Could you check a few things on this model? Use its own coordinates, in mm. Face numbers are marked on the shaded views. Give positions to 0.01 mm unless a question says otherwise; leave off trailing zeros. Write each question's results on one line, items separated by ' | '. Start each with the question number.
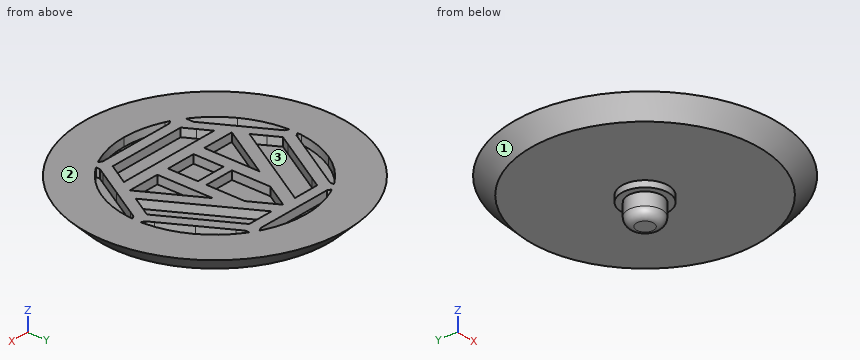
from build123d import *

# Parameters (mm, degrees)
F0_R     = 32
F1_DEPTH = 4
F3_R     = 5.5
F3_R_2   = 4.025
F4_DEPTH = 1.5
F5_DEPTH = 6.5
F7_DEPTH = 2
F8_R     = 2


# Not quite as in the source:
# - a fillet or chamfer that OpenCascade refuses, or shapes differently, is made with other operations: its cross-section is extruded or revolved along the edge and cut away or added


with BuildPart() as f1:
    # F0 (on Top) → F1 (new body)
    with BuildSketch(Plane.XY):
        Circle(F0_R)
    extrude(amount=F1_DEPTH)

    # F2: chamfer of 5 on 1 edges, made by hand

    # F2_s1 → F2_t2 (revolve, cut)
    with BuildSketch(Plane.XZ):
        Polygon((32, 5), (27, 0), (32, 0), align=None)
    revolve(axis=Axis((0, 0, 0), (0, 0, 1)), mode=Mode.SUBTRACT)

    # F3 (on face) → F4 (join)
    with BuildSketch(Plane(origin=(0, 0, 0), x_dir=(1, 0, 0), z_dir=(0, 0, -1))):
        Circle(F3_R)
        Circle(F3_R_2, mode=Mode.SUBTRACT)
    extrude(amount=F4_DEPTH)

    # F3 (on face) → F5 (join)
    with BuildSketch(Plane(origin=(0, 0, 0), x_dir=(1, 0, 0), z_dir=(0, 0, -1))):
        Circle(F3_R_2)
    extrude(amount=F5_DEPTH)

    # F6 (on face) → F7 (cut)
    with BuildSketch(Plane.XY.offset(4)):
        with BuildLine():
            Line((16.237976321, -9.375), (18.75, -10.8253175473))
            ThreePointArc((18.75, -10.8253175473), (20.6335015486, -6.5580952909), (21.5593108924, -1.9864827825))
            Line((21.5593108924, -1.9864827825), (19.9759526419, -2.9006350946))
            Line((19.9759526419, -2.9006350946), (16.237976321, -9.375))
        make_face()
        with BuildLine():
            ThreePointArc((12.5, -17.6776695297), (15.9962278967, -14.5900888646), (18.75, -10.8253175473))
            Line((18.75, -10.8253175473), (16.237976321, -9.375))
            Line((16.237976321, -9.375), (12.5, -15.8493649054))
            Line((12.5, -15.8493649054), (12.5, -17.6776695297))
        make_face()
        with BuildLine():
            ThreePointArc((21.5593108924, 1.9864827825), (20.6335020609, 6.5580936791), (18.7500016913, 10.8253146179))
            ThreePointArc((18.7500016913, 10.8253146179), (15.9962290364, 14.590087615), (12.5, 17.6776695297))
            Line((12.5, 17.6776695297), (12.5, 15.8493649054))
            Line((12.5, 15.8493649054), (16.2379763781, 9.3749999011))
            Line((16.2379763781, 9.3749999011), (19.9759526419, 2.9006350946))
            Line((19.9759526419, 2.9006350946), (21.5593108924, 1.9864827825))
        make_face()
        with BuildLine():
            ThreePointArc((9.0593108924, 19.6641523121), (4.6372736512, 21.1481841557), (-1.3e-09, 21.6506350946))
            ThreePointArc((-1.3e-09, 21.6506350946), (-4.6372736525, 21.1481841554), (-9.0593108924, 19.6641523121))
            Line((-9.0593108924, 19.6641523121), (-7.4759526419, 18.75))
            Line((-7.4759526419, 18.75), (-3.65e-08, 18.75))
            Line((-3.65e-08, 18.75), (7.4759526419, 18.75))
            Line((7.4759526419, 18.75), (9.0593108924, 19.6641523121))
        make_face()
        with BuildLine():
            ThreePointArc((-9.0593108924, -19.6641523121), (-4.6372736547, -21.1481841549), (-5.7e-09, -21.6506350946))
            ThreePointArc((-5.7e-09, -21.6506350946), (4.6372736491, -21.1481841562), (9.0593108924, -19.6641523121))
            Line((9.0593108924, -19.6641523121), (7.4759526419, -18.75))
            Line((7.4759526419, -18.75), (0, -18.75))
            Line((0, -18.75), (-7.4759526419, -18.75))
            Line((-7.4759526419, -18.75), (-9.0593108924, -19.6641523121))
        make_face()
        with BuildLine():
            ThreePointArc((11.6626587737, -18.2409536573), (12.0846117855, -17.9641909919), (12.5, -17.6776695297))
            Line((12.5, -17.6776695297), (12.5, -15.8493649054))
            Line((12.5, -15.8493649054), (11.6626587737, -17.2996824527))
            Line((11.6626587737, -17.2996824527), (11.6626587737, -18.2409536573))
        make_face()
        with BuildLine():
            Line((19.9759526419, -2.9006350946), (21.5593108924, -1.9864827825))
            ThreePointArc((21.5593108924, -1.9864827825), (21.5997516502, -1.4834853051), (21.6284586433, -0.979681945))
            Line((21.6284586433, -0.979681945), (20.8132938683, -1.4503175473))
            Line((20.8132938683, -1.4503175473), (19.9759526419, -2.9006350946))
        make_face()
        with BuildLine():
            ThreePointArc((21.6284586433, 0.979681945), (21.5997516502, 1.4834853051), (21.5593108924, 1.9864827825))
            Line((21.5593108924, 1.9864827825), (19.9759526419, 2.9006350946))
            Line((19.9759526419, 2.9006350946), (20.8132938683, 1.4503175473))
            Line((20.8132938683, 1.4503175473), (21.6284586433, 0.979681945))
        make_face()
        with BuildLine():
            Line((12.5, 15.8493649054), (12.5, 17.6776695297))
            ThreePointArc((12.5, 17.6776695297), (12.0846117855, 17.9641909919), (11.6626587737, 18.2409536573))
            Line((11.6626587737, 18.2409536573), (11.6626587737, 17.2996824527))
            Line((11.6626587737, 17.2996824527), (12.5, 15.8493649054))
        make_face()
        with BuildLine():
            ThreePointArc((-12.5, 17.6776695297), (-15.9962290427, 14.5900876082), (-18.7500017006, 10.8253146018))
            ThreePointArc((-18.7500017006, 10.8253146018), (-20.6335020637, 6.5580936703), (-21.5593108924, 1.9864827825))
            Line((-21.5593108924, 1.9864827825), (-19.9759526419, 2.9006350946))
            Line((-19.9759526419, 2.9006350946), (-16.2379762959, 9.3750000433))
            Line((-16.2379762959, 9.3750000433), (-12.5, 15.8493649054))
            Line((-12.5, 15.8493649054), (-12.5, 17.6776695297))
        make_face()
        with BuildLine():
            ThreePointArc((9.9657998697, 19.2206356023), (9.5151398647, 19.447676297), (9.0593108924, 19.6641523121))
            Line((9.0593108924, 19.6641523121), (7.4759526419, 18.75))
            Line((7.4759526419, 18.75), (9.1506350946, 18.75))
            Line((9.1506350946, 18.75), (9.9657998697, 19.2206356023))
        make_face()
        with BuildLine():
            Line((-7.4759526419, 18.75), (-9.0593108924, 19.6641523121))
            ThreePointArc((-9.0593108924, 19.6641523121), (-9.5151398647, 19.447676297), (-9.9657998697, 19.2206356023))
            Line((-9.9657998697, 19.2206356023), (-9.1506350946, 18.75))
            Line((-9.1506350946, 18.75), (-7.4759526419, 18.75))
        make_face()
        with BuildLine():
            Line((-16.237976321, -9.375), (-18.75, -10.8253175473))
            ThreePointArc((-18.75, -10.8253175473), (-15.9962278967, -14.5900888646), (-12.5, -17.6776695297))
            Line((-12.5, -17.6776695297), (-12.5, -15.8493649054))
            Line((-12.5, -15.8493649054), (-16.237976321, -9.375))
        make_face()
        with BuildLine():
            ThreePointArc((-21.5593108924, -1.9864827825), (-20.6335015486, -6.5580952909), (-18.75, -10.8253175473))
            Line((-18.75, -10.8253175473), (-16.237976321, -9.375))
            Line((-16.237976321, -9.375), (-19.9759526419, -2.9006350946))
            Line((-19.9759526419, -2.9006350946), (-21.5593108924, -1.9864827825))
        make_face()
        with BuildLine():
            ThreePointArc((-9.9657998697, -19.2206356023), (-9.5151398647, -19.447676297), (-9.0593108924, -19.6641523121))
            Line((-9.0593108924, -19.6641523121), (-7.4759526419, -18.75))
            Line((-7.4759526419, -18.75), (-9.1506350946, -18.75))
            Line((-9.1506350946, -18.75), (-9.9657998697, -19.2206356023))
        make_face()
        with BuildLine():
            Line((7.4759526419, -18.75), (9.0593108924, -19.6641523121))
            ThreePointArc((9.0593108924, -19.6641523121), (9.5151398647, -19.447676297), (9.9657998697, -19.2206356023))
            Line((9.9657998697, -19.2206356023), (9.1506350946, -18.75))
            Line((9.1506350946, -18.75), (7.4759526419, -18.75))
        make_face()
        Polygon((6.4743649054, -16.237976321), (9.375, -16.237976321), (10.8253175473, -13.7259526419), align=None)
        Polygon((17.2996824527, -2.512023679), (18.75, 0), (17.2996824527, 2.512023679), align=None)
        with BuildLine():
            ThreePointArc((-11.6626587737, 18.2409536573), (-12.0846117855, 17.9641909919), (-12.5, 17.6776695297))
            Line((-12.5, 17.6776695297), (-12.5, 15.8493649054))
            Line((-12.5, 15.8493649054), (-11.6626587737, 17.2996824527))
            Line((-11.6626587737, 17.2996824527), (-11.6626587737, 18.2409536573))
        make_face()
        with BuildLine():
            Line((-19.9759526419, 2.9006350946), (-21.5593108924, 1.9864827825))
            ThreePointArc((-21.5593108924, 1.9864827825), (-21.5997516502, 1.4834853051), (-21.6284586433, 0.979681945))
            Line((-21.6284586433, 0.979681945), (-20.8132938683, 1.4503175473))
            Line((-20.8132938683, 1.4503175473), (-19.9759526419, 2.9006350946))
        make_face()
        with BuildLine():
            ThreePointArc((-21.6284586433, -0.979681945), (-21.5997516502, -1.4834853051), (-21.5593108924, -1.9864827825))
            Line((-21.5593108924, -1.9864827825), (-19.9759526419, -2.9006350946))
            Line((-19.9759526419, -2.9006350946), (-20.8132938683, -1.4503175473))
            Line((-20.8132938683, -1.4503175473), (-21.6284586433, -0.979681945))
        make_face()
        Polygon((0, -16.237976321), (6.4743649054, -16.237976321), (10.8253175473, -13.7259526419), (12.4439087737, -10.9224704012), (-12.4439087737, -10.9224704012), (-10.8253175473, -13.7259526419), (-6.4743649054, -16.237976321), align=None)
        Polygon((15.6810912263, -5.3155059198), (17.2996824527, -2.512023679), (17.2996824527, 2.512023679), (10.8253175473, 13.7259526419), (6.4743649054, 16.237976321), (3.2371824527, 16.237976321), align=None)
        Polygon((-17.2996824527, 2.512023679), (-18.75, 0), (-17.2996824527, -2.512023679), align=None)
        Polygon((-10.8253175473, -13.7259526419), (-9.375, -16.237976321), (-6.4743649054, -16.237976321), align=None)
        Polygon((-7.03125, 4.0594940802), (-14.0625, -8.1189881605), (-6.4743649054, -8.1189881605), (-6.4743649054, 5.0240473581), align=None)
        Polygon((10.8253175473, 13.7259526419), (9.375, 16.237976321), (6.4743649054, 16.237976321), align=None)
        Polygon((-6.4743649054, 16.237976321), (-9.375, 16.237976321), (-10.8253175473, 13.7259526419), align=None)
        Polygon((-10.8253175473, 13.7259526419), (-17.2996824527, 2.512023679), (-17.2996824527, -2.512023679), (-15.6810912263, -5.3155059198), (-3.2371824527, 16.237976321), (-6.4743649054, 16.237976321), align=None)
        Polygon((6.4743649054, -8.1189881605), (14.0625, -8.1189881605), (7.03125, 4.0594940802), (6.4743649054, 5.0240473581), align=None)
        Polygon((-3.515625, -4.0594940802), (-3.515625, -8.1189881605), (3.515625, -8.1189881605), (3.515625, -1.0148735201), (0, -1.0148735201), (-3.515625, -1.0148735201), (-3.515625, -2.0297470401), align=None)
        Polygon((3.515625, 10.1487352006), (0, 16.237976321), (-3.515625, 10.1487352006), (-3.515625, 1.0148735201), (0, 1.0148735201), (3.515625, 1.0148735201), align=None)
    extrude(amount=-F7_DEPTH, mode=Mode.SUBTRACT)

    # F8
    f8_edges = [f1.edges().sort_by_distance(p)[0] for p in [
        (-4.025, 0, -6.5),
    ]]
    fillet(f8_edges, radius=F8_R)


solid = f1.part
Q1. If we section it at A-A (z = 2.75): Count the separate pieces of the cut face and the enclosed holes in it, plus the area to 3 significant figures.
Q2. If we mould it in two halves opening along Y, with no side actions, what happens to the marked faces 1, 2 and 3? For each: pulls with the +Y half, pulls with the -Y half, needs draft (parallel to the pull), parting line crosses it, or undercut.
Q3. Please list where these lines run through material, in increasing order: line 1 (Y direction, x = 9, z = 2.5); line 2 (X direction, y = 15.5, z = 3.5); line 3 (X direction, y = -3.5, z = -4.25). Write a range as [from, to].
Q4. I'm going to push flat-ended pins straight in: P1, Ø0.6, axis at x = -0.5, z = 2.5, coming from the -Y side; P2, Ø0.6, axis at x = -7.5, z = 3, coming from the -Y side; P3, Ø5, axis at y = -7.5, z = -1.5, coming from the +X side; P4, Ø7.5, axis at x = -17.5, y = -11.5, coming from the +Z side. Where does each tip first touch, or does it pass through?
Determined:
1) separate pieces: 1 | enclosed holes: 13 | area: 1,950 mm²
2) face 1: parting line crosses it | face 2: needs draft | face 3: undercut
3) line 1: y = [-28.09, -19.69], [-18.75, -16.24], [-10.92, -8.12], [0.65, 6.26], [16.24, 18.75], [19.69, 28.09] | line 2: x = [-26.27, -15.12], [-12.7, -9.8], [-3.66, -0.43], [0.43, 3.66], [9.8, 12.7], [15.12, 26.27] | line 3: x = [-1.99, 1.99]
4) P1: stops at y = -29.8 | P2: stops at y = -29.37 | P3: stops at x = 27.06 | P4: stops at z = 4
